Geometry check sheet. Reference: the model listing, model coordinates, mm. A direction names the side the tool comes from. Round coordinates to 2 decimals unless told otherwise and drop trailing zeros. Loops run counter-clockwise (first coordinate to the right, second up) from the corner with the lowest first, then second, coordinate; pieces in that order, holes last. Notation, with made-up numbers: (25.5, -13.75) -> (69.5, -13.75) arc R19 ccw to (69.5, 13.25) -> close; hole circle Ø9 at (79, 68). An arc over 180 degrees is marked (long way). Use a Markdown table: item, result. Add a question column.
Q1. Sectioned sample at C-C, the plane z = 2.65. Enter the section's corners in (x, y) (3 decimals).
Q2. Sectioned sample at A-A, the plane x = 0. Enter the section's corners in (y, z) (3 decimals).
Q3. Sectioned sample at B-B, the plane y = -103.5. Enter the section's corners in (x, z).
Q4. Material ranges on L1, parallel to Y at x = 0, z = 2.95 (3 decimals); L2, parallel to X at y = -106, z = 1.95; L3, parallel to Y at x = -3.5, z = 2.2, recorded low to high.
Q5. Sectioned sample at D-D, the plane x = 17. Enter the section's corners in (y, z), then the cut area to 3 significant figures.
Q6. Set-up check for faces 1 (the face through (9, -98, 4)), 2 (the face through (5, -97, 2)): record each of +Z, -Z, +X, -X, +Y, -Y from which the full face is reachable in a straight line by a thin tool's end or side.
Q7. Release check for a two-part mould opening along X. For faces 3 (the face through (-5, -95, 2)), 4 (the face through (-20, -99, 2)), 5 (the face through (0, -220, 2)) record: released by +X, released by -X, zero draft, split by the parting line, or undercut.
```python
from build123d import *

# Parameters (mm, degrees)
SKETCH_1_R          = 8
EXTRUDE_1_DEPTH     = 4
CUT_EXTRUDE_2_DEPTH = 221.943431674


with BuildPart() as part:
    # 草图1 → 凸台-拉伸1 (new body)
    with BuildSketch(Plane.XY):
        with BuildLine():
            Line((-20, 0), (-20, -200))
            ThreePointArc((-20, -200), (0, -220), (20, -200))
            Line((20, -200), (20, 0))
            ThreePointArc((20, 0), (0, 20), (-20, 0))
        make_face()
        Circle(SKETCH_1_R, mode=Mode.SUBTRACT)
        with Locations((0, -200)):
            Circle(SKETCH_1_R, mode=Mode.SUBTRACT)
    extrude(amount=EXTRUDE_1_DEPTH)

    # 草图2 → 切除-拉伸2 (cut, through all)
    with BuildSketch(Plane.XY.offset(4)):
        with BuildLine():
            Line((-5, -31.845004689), (-5, -159.845004689))
            ThreePointArc((-5, -159.845004689), (0, -164.845004689), (5, -159.845004689))
            Line((5, -159.845004689), (5, -31.845004689))
            ThreePointArc((5, -31.845004689), (0, -26.845004689), (-5, -31.845004689))
        make_face()
    extrude(amount=-CUT_EXTRUDE_2_DEPTH, mode=Mode.SUBTRACT)


solid = part.part
```
Values:
| question | item | result |
|---|---|---|
| 1 | outline | (-20, -200) arc R20 ccw to (20, -200) -> (20, 0) arc R20 ccw to (-20, 0) -> close; hole circle Ø16 at (0, -200); hole circle Ø16 at (0, 0); hole (-5, -159.845) arc R5 ccw to (5, -159.845) -> (5, -31.845) arc R5 ccw to (-5, -31.845) -> close |
| 2 | outline | (-220, 0) -> (-208, 0) -> (-208, 4) -> (-220, 4) -> close; (-192, 0) -> (-164.845, 0) -> (-164.845, 4) -> (-192, 4) -> close; (-26.845, 0) -> (-8, 0) -> (-8, 4) -> (-26.845, 4) -> close; (8, 0) -> (20, 0) -> (20, 4) -> (8, 4) -> close |
| 3 | outline | (-20, 0) -> (-5, 0) -> (-5, 4) -> (-20, 4) -> close; (5, 0) -> (20, 0) -> (20, 4) -> (5, 4) -> close |
| 4 | L1 | -220 to -208, -192 to -164.845, -26.845 to -8, 8 to 20 |
| 4 | L2 | -20 to -5, 5 to 20 |
| 4 | L3 | -219.69 to -207.19, -192.81 to -163.42, -28.27 to -7.19, 7.19 to 19.69 |
| 5 | outline | (-210.54, 0) -> (10.54, 0) -> (10.54, 4) -> (-210.54, 4) -> close |
| 5 | area | 884 mm^2 |
| 6 | face 1 | +Z, +X, -X, +Y, -Y |
| 6 | face 2 | +Z, -Z |
| 7 | face 3 | undercut |
| 7 | face 4 | released by -X |
| 7 | face 5 | split by the parting line |
